from build123d import *

# Parameters (mm, degrees)
SKETCH1_R           = 11.25
SKETCH3_R           = 11.25
SKETCH3_5_R         = 12.25
BOSS_EXTRUDE1_DEPTH = 0.5
SKETCH1_4_R         = 12.25
BOSS_EXTRUDE2_DEPTH = 0.5


with BuildPart() as part:
    # Sketch1 → Loft1 section 0
    with BuildSketch(Plane.XY):
        Circle(SKETCH1_R)
    # Sketch3 → Loft1 section 1
    with BuildSketch(Plane(origin=(0, -2.247482777, 5.854892806), x_dir=(1, 0, 0), z_dir=(0, -0.358367949545301, 0.9335804264972015))):
        with Locations((0, 2.407379925)):
            Circle(SKETCH3_R)
    loft()

    # Sketch3<5> → Boss-Extrude1 (add)
    with BuildSketch(Plane(origin=(0, -2.247482777, 5.854892806), x_dir=(1, 0, 0), z_dir=(0, -0.358367949545301, 0.9335804264972015))):
        with Locations(Location((0, 2.407379925, 0), (0, 0, 270))):
            Circle(SKETCH3_5_R)
    extrude(amount=-BOSS_EXTRUDE1_DEPTH)

    # Sketch1<4> → Boss-Extrude2 (add)
    with BuildSketch(Plane.XY):
        Circle(SKETCH1_4_R)
    extrude(amount=BOSS_EXTRUDE2_DEPTH)


solid = part.part
Can you work these out from the model? Positions are in its coordinate system, mm. Round coordinates to 2 decimals unless told otherwise and drop trailing zeros. Write each question's results on one line, items separated by ' | '. Start each with the question number.
1) Please list where these lines run through material, in increasing order: line 1 (X direction, y = 1.5, z = 5); line 2 (X direction, y = 7.75, z = 8); line 3 (Z direction, x = -7.75, y = -5).
2) For pin 1 Ø5 at (y, z) = (-9, 8) entering from -X; pin 2 Ø6 at (x, y) = (-10, 4) entering from -Z; pin 3 Ø1 at (x, z) = (5.5, 7) entering from +Y; pin 4 Ø2 at (y, z) = (4, 5) entering from +X, each with a flat end and sliding along its axis, tell me the tip position at first contact or that it passes through.
3) We'd pull the mould along Y, two halves only. Please class faces 1 (the cylindrical face through (10.3, -6.1, 4.1)), 2 (the flat face through (0.17, 0.16, 6.78)), 3 (the flat face through (3, -11, 0.5)), 4 (the flat face through (2.779, 10.398, 10.174)): released by +Y, released by -Y, zero draft, split by the parting line, or undercut.
Here are the results:
1) line 1: x = -11.14 to 11.14 | line 2: x = -7.7 to 7.7 | line 3: z = 0 to 4.8
2) pin 1: passes through | pin 2: stops at z = 0 | pin 3: stops at y = 9.63 | pin 4: stops at x = 10.81
3) face 1: split by the parting line | face 2: released by -Y | face 3: zero draft | face 4: undercut
